For this review, use the dimensioned drawing (mm, ordinates from the lowest corner) and the shaded views. A direction names the side the tool comes from. Round coordinates to 2 decimals unless told otherwise and drop trailing zeros. Order: outer loops, then holes, each group sorted by start corner. A loop starts at its lowest first (then second) coordinate and runs counter-clockwise, first axis right, second up. Notation, with made-up numbers: M -1,52 L 46,52 A12 cw 46,56 Z; hole C 55.5,2 d7. An arc over 180 degrees is marked long. Put each result on its own line as item: value.
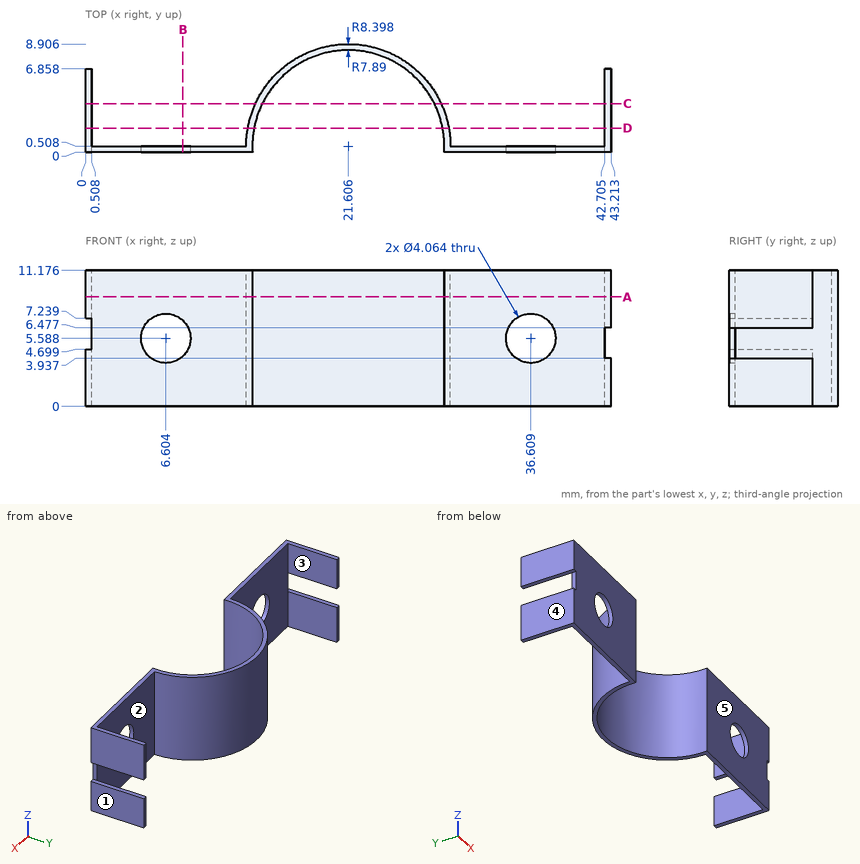
(1) To check wall thickness, follow L1, parallel to X at y = 3.75, z = 0.75 (1 decimal); L2, parallel to X at y = 3, z = 2 (1 decimal); L3, parallel to X at y = 3.75, z = 6.75 (1 decimal). State the ranges of each line that lie inside material, in increasing order.
A:
L1: x = 0 to 0.5, 13.9 to 14.4, 28.8 to 29.4, 42.7 to 43.2
L2: x = 0 to 0.5, 13.6 to 14.1, 29.1 to 29.6, 42.7 to 43.2
L3: x = 13.9 to 14.4, 28.8 to 29.4, 42.7 to 43.2
(2) For the marked faces 1 and 2, list the 3-axis set-ups (+Z, -Z, +X, -X, +Y, -Y) from which the entire face can be reached by the end or side of a thin tool; tool diameter is ignored.
A:
face 1: +Z, -Z, +X, +Y, -Y
face 2: +Z, -Z, +Y
(3) Add section C-C on y = 4. Give the boundary of the cut face in (x, z) (1 decimal).
A:
outline: M 0,0 L 0.5,0 L 0.5,4.7 L 0,4.7 Z; M 0,7.2 L 0.5,7.2 L 0.5,11.2 L 0,11.2 Z; M 14,0 L 14.5,0 L 14.5,11.2 L 14,11.2 Z; M 28.7,0 L 29.2,0 L 29.2,11.2 L 28.7,11.2 Z; M 42.7,0 L 43.2,0 L 43.2,3.9 L 42.7,3.9 Z; M 42.7,6.5 L 43.2,6.5 L 43.2,11.2 L 42.7,11.2 Z
(4) Add section D-D on y = 2. Give the boundary of the cut face in (x, z) (1 decimal).
A:
outline: M 0,0 L 0.5,0 L 0.5,4.7 L 0,4.7 Z; M 0,7.2 L 0.5,7.2 L 0.5,11.2 L 0,11.2 Z; M 13.3,0 L 13.9,0 L 13.9,11.2 L 13.3,11.2 Z; M 29.4,0 L 29.9,0 L 29.9,11.2 L 29.4,11.2 Z; M 42.7,0 L 43.2,0 L 43.2,3.9 L 42.7,3.9 Z; M 42.7,6.5 L 43.2,6.5 L 43.2,11.2 L 42.7,11.2 Z
(5) Add section B-B on x = 8. Give the boundary of the cut face in (y, z) (1 decimal).
A:
outline: M 0,0 L 0.5,0 L 0.5,4.1 L 0,4.1 Z; M 0,7.1 L 0.5,7.1 L 0.5,11.2 L 0,11.2 Z
(6) Add section A-A on z = 9. Give the boundary of the cut face in (x, y) (1 decimal).
A:
outline: M 0,0 L 13.7,0 A7.9 cw long 29.5,0 L 43.2,0 L 43.2,6.9 L 42.7,6.9 L 42.7,0.5 L 30,0.5 A8.4 ccw 13.2,0.5 L 0.5,0.5 L 0.5,6.9 L 0,6.9 Z
(7) Draft analysis for pull direction X (two halves, no side actions). For the marked faces 3, 4 and 5, state which applies: released by +X, released by -X, zero draft, split by the parting line, or undercut.
A:
face 3: undercut
face 4: released by -X
face 5: zero draft
(8) Insertion check: pin 1 Ø1 at (x, z) = (10, 7.5) entering from +Y; pin 2 Ø1.5 at (y, z) = (6, 4) entering from -X; pin 3 Ø1.5 at (x, z) = (27, 2.5) entering from +Y (1 decimal). Each pin has a flat end and moves straight along its axis. Give the tip position at first contact, or say it passes through.
A:
pin 1: stops at y = 0.51
pin 2: stops at x = 0
pin 3: stops at y = 7.5
